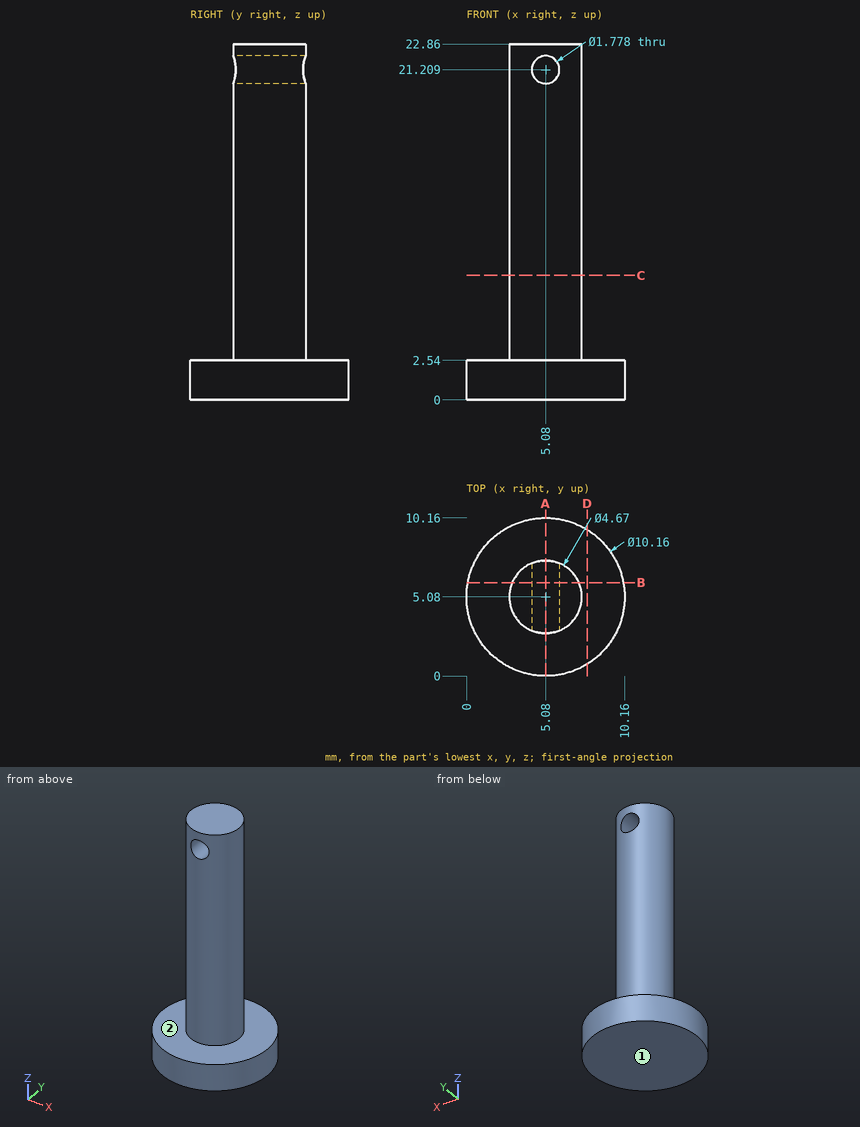
For this review, use the dimensioned drawing (mm, ordinates from the lowest corner) and the shaded views. A direction names the side the tool comes from. Give positions to 0.01 mm unless a question says otherwise; leave off trailing zeros. Order: outer loops, then holes, each group sorted by start corner. A loop starts at its lowest first (then second) coordinate and runs counter-clockwise, first axis right, second up. Notation, with made-up numbers: (68.5, 71) - (82.5, 71) arc R10 cw to (82.5, 78) - close; hole circle Ø5 at (83.5, 15.5). An arc over 180 degrees is marked (long way). Use a Markdown table: item, result. Add a question column.
(1) Add section A-A on x = 5.08. Give the boundary of the cut face in (y, z) (3 decimals).
(2) Add section D-D on x = 7.75. Give the boundary of the cut face in (y, z), then the cut area to 3 significant figures.
(3) Machinability: for the marked faces 1 and 2, which of the approach directions +Z, -Z, +X, -X, +Y, -Y give a long, thin tool a straight path to every point of the face, cutting with its end or side? Answer none if there is none.
(4) Add section C-C on z = 8. Give the boundary of the cut face in (x, y) (3 decimals), then the cut area to 3 significant figures.
(5) Add section B-B on y = 6. Give the boundary of the cut face in (x, z), then the cut area to 3 significant figures.
(6) Wall thickness on probe 1 along Z at (x, y) = (5.08, 4.1); probe 2 along Z at (x, y) = (5, 1); probe 3 along X at (y, z) = (5.5, 19.25): over which ranges is each line inside the solid? List them lowest first. Write a range as [from, to].
(7) Clearance check with flat-ended pins moving along their axes: P1, Ø6, axis at y = 5, z = 15, coming from the +X side (3 decimals); P2, Ø2, axis at x = 5.08, z = 21.209, coming from the -Y side (3 decimals); P3, Ø2, axis at x = 7, z = 16, coming from the -Y side. State where each tip first meets the part, or that it passes through.
Report:
| question | item | result |
|---|---|---|
| 1 | outline | (0, 0) - (10.16, 0) - (10.16, 2.54) - (7.415, 2.54) - (7.415, 20.32) - (2.745, 20.32) - (2.745, 2.54) - (0, 2.54) - close; (2.745, 22.098) - (7.415, 22.098) - (7.415, 22.86) - (2.745, 22.86) - close |
| 2 | outline | (0.76, 0) - (9.4, 0) - (9.4, 2.54) - (0.76, 2.54) - close |
| 2 | area | 22.0 mm² |
| 3 | face 1 | -Z, +X, -X, +Y, -Y |
| 3 | face 2 | +Z |
| 4 | outline | circle Ø4.67 at (5.08, 5.08) |
| 4 | area | 17.1 mm² |
| 5 | outline | (0.08, 0) - (10.08, 0) - (10.08, 2.54) - (7.23, 2.54) - (7.23, 22.86) - (2.93, 22.86) - (2.93, 2.54) - (0.08, 2.54) - close; hole circle Ø1.78 at (5.08, 21.21) |
| 5 | area | 110 mm² |
| 6 | probe 1 | z = [0, 20.32], [22.1, 22.86] |
| 6 | probe 2 | z = [0, 2.54] |
| 6 | probe 3 | x = [2.78, 7.38] |
| 7 | P1 | stops at x = 7.415 |
| 7 | P2 | stops at y = 2.745 |
| 7 | P3 | stops at y = 2.93 |
